from build123d import *

# Parameters (mm, degrees)
F1_DEPTH = 380
F2_R     = 25
F3_DEPTH = 10
F4_R     = 12.5
F5_DEPTH = 10


with BuildPart() as f1:
    # F0 (on Front) → F1 (new body)
    with BuildSketch(Plane.XZ):
        with BuildLine():
            Line((-290, -187.5), (290, -187.5))
            ThreePointArc((290, -187.5), (325.355339, -172.855339), (340, -137.5))
            Line((340, -137.5), (340, 137.5))
            ThreePointArc((340, 137.5), (325.355339, 172.855339), (290, 187.5))
            Line((290, 187.5), (-290, 187.5))
            ThreePointArc((-290, 187.5), (-325.355339, 172.855339), (-340, 137.5))
            Line((-340, 137.5), (-340, -137.5))
            ThreePointArc((-340, -137.5), (-325.355339, -172.855339), (-290, -187.5))
        make_face()
        with BuildLine():
            ThreePointArc((315, -137.5), (307.67767, -155.17767), (290, -162.5))
            Line((290, -162.5), (-290, -162.5))
            ThreePointArc((-290, -162.5), (-307.67767, -155.17767), (-315, -137.5))
            Line((-315, -137.5), (-315, 137.5))
            ThreePointArc((-315, 137.5), (-307.67767, 155.17767), (-290, 162.5))
            Line((-290, 162.5), (290, 162.5))
            ThreePointArc((290, 162.5), (307.67767, 155.17767), (315, 137.5))
            Line((315, 137.5), (315, -137.5))
        make_face(mode=Mode.SUBTRACT)
    extrude(amount=F1_DEPTH)

    # F2 (on face) → F3 (cut)
    with BuildSketch(Plane(origin=(0, 0, -187.5), x_dir=(1, 0, 0), z_dir=(0, 0, -1))):
        with Locations((-240, 330)):
            Circle(F2_R)
        with Locations((-240, 50)):
            Circle(F2_R)
        with Locations((240, 50)):
            Circle(F2_R)
        with Locations((240, 330)):
            Circle(F2_R)
    extrude(amount=-F3_DEPTH, mode=Mode.SUBTRACT)

    # F4 (on face) → F5 (cut)
    with BuildSketch(Plane.XY.offset(187.5)):
        with Locations((-240, -330)):
            Circle(F4_R)
        with Locations((-240, -50)):
            Circle(F4_R)
        with Locations((0, -330)):
            Circle(F4_R)
        with Locations((0, -50)):
            Circle(F4_R)
        with Locations((240, -330)):
            Circle(F4_R)
        with Locations((240, -50)):
            Circle(F4_R)
    extrude(amount=-F5_DEPTH, mode=Mode.SUBTRACT)


solid = f1.part
Read the model definition and answer for the solid it produces. Units are mm, in the model's axes. A direction names the side the tool comes from. Round coordinates to 2 decimals unless told otherwise and drop trailing zeros. Write each loop counter-clockwise with the first axis right and the second up, starting at its lowest first coordinate (ties: lowest second). Pieces come first, ordered by that corner, then holes.
Q1. Find section D-D on x = 0. Determine the outline of the cut face in (y, z), and give its area (3 significant figures).
Values:
outline: (-380, -187.5) - (0, -187.5) - (0, -162.5) - (-380, -162.5) - close; (-380, 162.5) - (0, 162.5) - (0, 187.5) - (-37.5, 187.5) - (-37.5, 177.5) - (-62.5, 177.5) - (-62.5, 187.5) - (-317.5, 187.5) - (-317.5, 177.5) - (-342.5, 177.5) - (-342.5, 187.5) - (-380, 187.5) - close
area: 18,500 mm2
Q2. Find section C-C on y = -160.5. Determine the outline of the cut face in (x, z).
Values:
outline: (-340, -137.5) arc R50 ccw to (-290, -187.5) - (290, -187.5) arc R50 ccw to (340, -137.5) - (340, 137.5) arc R50 ccw to (290, 187.5) - (-290, 187.5) arc R50 ccw to (-340, 137.5) - close; hole (-315, -137.5) arc R25 ccw to (-290, -162.5) - (290, -162.5) arc R25 ccw to (315, -137.5) - (315, 137.5) arc R25 ccw to (290, 162.5) - (-290, 162.5) arc R25 ccw to (-315, 137.5) - close
Q3. Find section A-A on x = -240. Determine the outline of the cut face in (y, z), and give its area (3 significant figures).
Values:
outline: (-380, -187.5) - (-355, -187.5) - (-355, -177.5) - (-305, -177.5) - (-305, -187.5) - (-75, -187.5) - (-75, -177.5) - (-25, -177.5) - (-25, -187.5) - (0, -187.5) - (0, -162.5) - (-380, -162.5) - close; (-380, 162.5) - (0, 162.5) - (0, 187.5) - (-37.5, 187.5) - (-37.5, 177.5) - (-62.5, 177.5) - (-62.5, 187.5) - (-317.5, 187.5) - (-317.5, 177.5) - (-342.5, 177.5) - (-342.5, 187.5) - (-380, 187.5) - close
area: 17,500 mm2
Q4. The mould has two halves that part along X. Classify faces 5 (the face through (240, -330, -177.5)), 6 (the face through (-27, 0, -166)), 7 (the face through (325.742, -187.34, 172.464)): released by +X, released by -X, zero draft, split by the parting line, or undercut.
Values:
face 5: undercut
face 6: zero draft
face 7: released by +X
Q5. Straight lines are drawn through the part: line 1 (X direction, y = -257.5, z = 61); line 2 (Z direction, x = -132, y = -21); line 3 (Z direction, x = -248.5, y = -312.5). For each, find the intervals that lie inside material, in ascending order.
Values:
line 1: x = -340 to -315, 315 to 340
line 2: z = -187.5 to -162.5, 162.5 to 187.5
line 3: z = -177.5 to -162.5, 162.5 to 187.5
Q6. Flat-ended cylindrical pins translate along their axes: P1, Ø12.5, axis at x = 234.5, y = -56, coming from the +Z side; P2, Ø15, axis at x = 240, y = -50, coming from the +Z side; P3, Ø20, axis at x = -240, y = -330, coming from the -Z side. Find the tip coordinate at first contact, or state that the pin passes through.
Values:
P1: stops at z = 187.5
P2: stops at z = 177.5
P3: stops at z = -177.5
Q7. A tool of negligible diameter and unlimited length cuts with its end or side. For faces 1 (the face through (-240, -50, -177.5)), 2 (the face through (4, -187, 187.5)), 3 (the face through (-240, -50, 177.5)), 4 (the face through (-307.482, -187.34, -155.371)), from which of +Z, -Z, +X, -X, +Y, -Y can it reach the whole face along a straight path? Write none if from no direction.
Values:
face 1: -Z
face 2: +Z, +X, -X, +Y, -Y
face 3: +Z
face 4: +Y, -Y
Q8. Find section B-B on z = -85.5. Determine the outline of the cut face in (x, y).
Values:
outline: (-340, -380) - (-315, -380) - (-315, 0) - (-340, 0) - close; (315, -380) - (340, -380) - (340, 0) - (315, 0) - close
